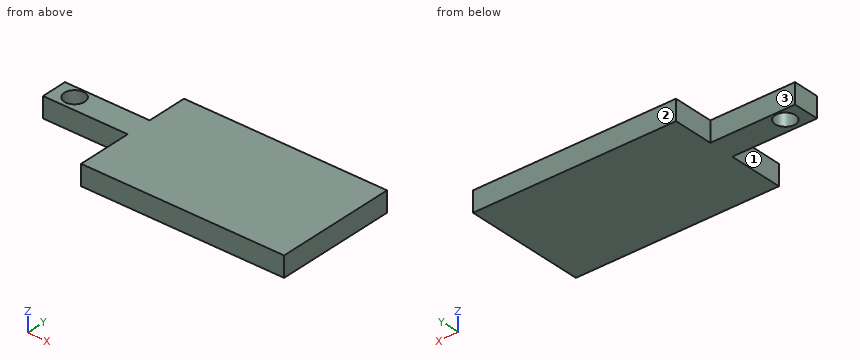
```python
from build123d import *

# Parameters (mm, degrees)
F0_W     = 106.009863
F0_H     = 32.523151
F1_DEPTH = 25.4
F2_R     = 12.7
F3_DEPTH = 25.4


with BuildPart() as f1:
    # F0 (on Top) → F1 (new body)
    with BuildSketch(Plane.XY):
        Polygon((0, 69.076849), (0, 0), (254, 0), (254, 152.4), (0, 152.4), (0, 101.6), align=None)
        with Locations((-53.004931, 85.338425)):
            Rectangle(F0_W, F0_H)
    extrude(amount=F1_DEPTH)

    # F2 (on face) → F3 (cut)
    with BuildSketch(Plane.XY.offset(25.4)):
        with Locations((-81.52055, 86.884722)):
            Circle(F2_R)
    extrude(amount=-F3_DEPTH, mode=Mode.SUBTRACT)


solid = f1.part
```
Input: part model. Units: mm. Frame: model coordinates. Face numbers are marked on the shaded views. A direction names the side the tool comes from. Coordinates: 2 decimals unless noted, no trailing zeros. Loops run counter-clockwise (first coordinate to the right, second up) from the corner with the lowest first, then second, coordinate; pieces in that order, holes last.
Q1. Section A-A, the plane z = 6. Return the cut outline in (x, y).
Results are:
outline: (-106.01, 69.08) - (0, 69.08) - (0, 0) - (254, 0) - (254, 152.4) - (0, 152.4) - (0, 101.6) - (-106.01, 101.6) - close; hole circle Ø25.4 at (-81.52, 86.88)
Q2. Section B-B, the plane y = 93.5. Return the cut outline in (x, z).
Results are:
outline: (-106.01, 0) - (-92.36, 0) - (-92.36, 25.4) - (-106.01, 25.4) - close; (-70.68, 0) - (254, 0) - (254, 25.4) - (-70.68, 25.4) - close
Q3. Section C-C, the plane x = -42.5. Return the cut outline in (y, z).
Results are:
outline: (69.08, 0) - (101.6, 0) - (101.6, 25.4) - (69.08, 25.4) - close
Q4. Contact query for flat-ended pins moving along their axis: pin 1 (1.5 mm diameter, centred on y = 111, z = 7, fed in from -X); pin 2 (12.5 mm diameter, centred on x = -65.5, z = 13, fed in from -Y). Output: stop coordinate, or through.
Results are:
pin 1: stops at x = 0
pin 2: stops at y = 69.08
Q5. Line query: line 1 along X through (y, z) = (40, 17.5); line 2 along Y through (x, z) = (-40, 3.75); line 3 along Y through (x, z) = (-80, 14). Output: solid intervals per line, ascending.
Results are:
line 1: x = 0 to 254
line 2: y = 69.08 to 101.6
line 3: y = 69.08 to 74.28, 99.49 to 101.6
Q6. Section D-D, the plane y = 114.5. Return the cut outline in (x, z), and give its area (3 significant figures).
Results are:
outline: (0, 0) - (254, 0) - (254, 25.4) - (0, 25.4) - close
area: 6,450 mm2
Q7. Set-up query: the marked faces 1, 2 and 3. Return all of +Z, -Z, +X, -X, +Y, -Y with unobstructed straight access to the full face (end or side cutting, diameter ignored); none if empty.
Results are:
face 1: +Z, -Z, -X, -Y
face 2: +Z, -Z, +X, -X, +Y
face 3: +Z, -Z, -X, +Y
